```python
from build123d import *


with BuildPart() as part:
    # Sketch → Revolution (revolve)
    with BuildSketch(Plane.XZ):
        with BuildLine():
            Line((-32.5, 0), (-32.5, 5))
            ThreePointArc((-32.3, 5.2), (-32.441421, 5.141421), (-32.5, 5))
            Line((-32.3, 5.2), (-31, 5.2))
            Line((-31, 5.2), (-31, 6.2))
            Line((-31, 6.2), (-32, 6.2))
            Line((-32, 6.2), (-32, 8))
            ThreePointArc((-31, 9), (-31.707107, 8.707107), (-32, 8))
            Line((-31, 9), (-30, 9))
            ThreePointArc((-30, 9), (-29.5, 8.866025), (-29, 9))
            Line((-29, 9), (31.5, 9))
            ThreePointArc((32.5, 8), (32.207107, 8.707107), (31.5, 9))
            Line((32.5, 8), (32.5, 0))
            Line((32.5, 0), (-32.5, 0))
        make_face()
    revolve(axis=Axis((0, 0, 0), (1, 0, 0)))


solid = part.part
```
Geometry: final body of the model. Coordinates: model frame, mm. A direction names the side the tool comes from. Round coordinates to 2 decimals unless told otherwise and drop trailing zeros. Loops run counter-clockwise (first coordinate to the right, second up) from the corner with the lowest first, then second, coordinate; pieces in that order, holes last. Notation, with made-up numbers: (62, -30) -> (85, -30) arc R26 cw to (85, 9) -> close; hole circle Ø1 at (76, 26). An arc over 180 degrees is marked (long way). Use one line per item in the form item = value. Start each with the question number.
1) Line query: L1, parallel to Z at x = -31.4, y = 0; L2, parallel to Y at x = -31.45, z = 0; L3, parallel to Y at x = -31.15, z = 0. Output: solid intervals per line, ascending.
2) Section A-A on x = 28.5. Output: boundary loops of the cut face in (y, z).
3) First-contact query: P1, Ø2, axis at x = -10, y = 4, coming from the -Z side; P2, Ø3, axis at x = -25.5, y = 5.5, coming from the -Z side; P3, Ø1.5, axis at x = -5.5, z = -6.5, coming from the +Y side. Flat tips, straight axial feed; report the tip coordinate or a pass-through.
4) Draft query along Z for faces 1 (the cylindrical face through (-31.641, -5.156, -0.677)), 2 (the cylindrical face through (-30.493, -8.923, -1.172)), 3 (the flat face through (-32.5, 0, 0)). Return one class per face: released by +Z, released by -Z, zero draft, split by the parting line, or undercut.
5) Access query for faces 4 (the cylindrical face through (1.674, -8.923, -1.172)), 5 (the cylindrical face through (-31.51, 5.5, 2.86)). Directions: +Z, -Z, +X, -X, +Y, -Y. A direction counts if a zero-diameter tool reaches every point of the face in a straight line with its end or side. Return the directions, or none.
Response:
q1.L1 = -8.92 to -6.2, -5.2 to 5.2, 6.2 to 8.92
q1.L2 = -8.89 to -6.2, -5.2 to 5.2, 6.2 to 8.89
q1.L3 = -8.99 to -6.2, -5.2 to 5.2, 6.2 to 8.99
q2.outline = circle Ø18 at (0, 0)
q3.P1 = -8.49
q3.P2 = -8.06
q3.P3 = 6.92
q4.face_1 = undercut
q4.face_2 = split by the parting line
q4.face_3 = zero draft
q5.face_4 = +X, -X
q5.face_5 = -X
